Geometry: see drawing. Coordinates: mm, zero at the bounding-box minimum. Give positions to 0.01 mm unless a question says otherwise; leave off trailing zeros. Write each loop counter-clockwise with the first axis right and the second up, starting at its lowest first coordinate (ties: lowest second). Pieces come first, ordered by that corner, then holes. Notation, with made-up numbers: (-36, 10) - (-26, 10) arc R21 ccw to (-26, 43) - close; hole circle Ø1 at (7, -5). An arc over 180 degrees is marked (long way). Use a Markdown table: item, result. Add a question column.
1. Pin query (flat end, axial travel): pin 1 (3 mm diameter, centred on y = 86, z = 2, fed in from -X). Return the tip coordinate at first contact, or that it passes through.
2. Material intervals for probe 1 along X at (y, z) = (81.5, 5.5); probe 2 along Y at (x, z) = (42, 3.5) (1 decimal); probe 3 along X at (y, z) = (75, 6.25) (1 decimal), sorted ascending.
3. Section query A-A, the plane y = 79.5. Return loops of the section in (x, z).
4. Section query C-C, the plane z = 4.5. Return loops of the section in (x, y).
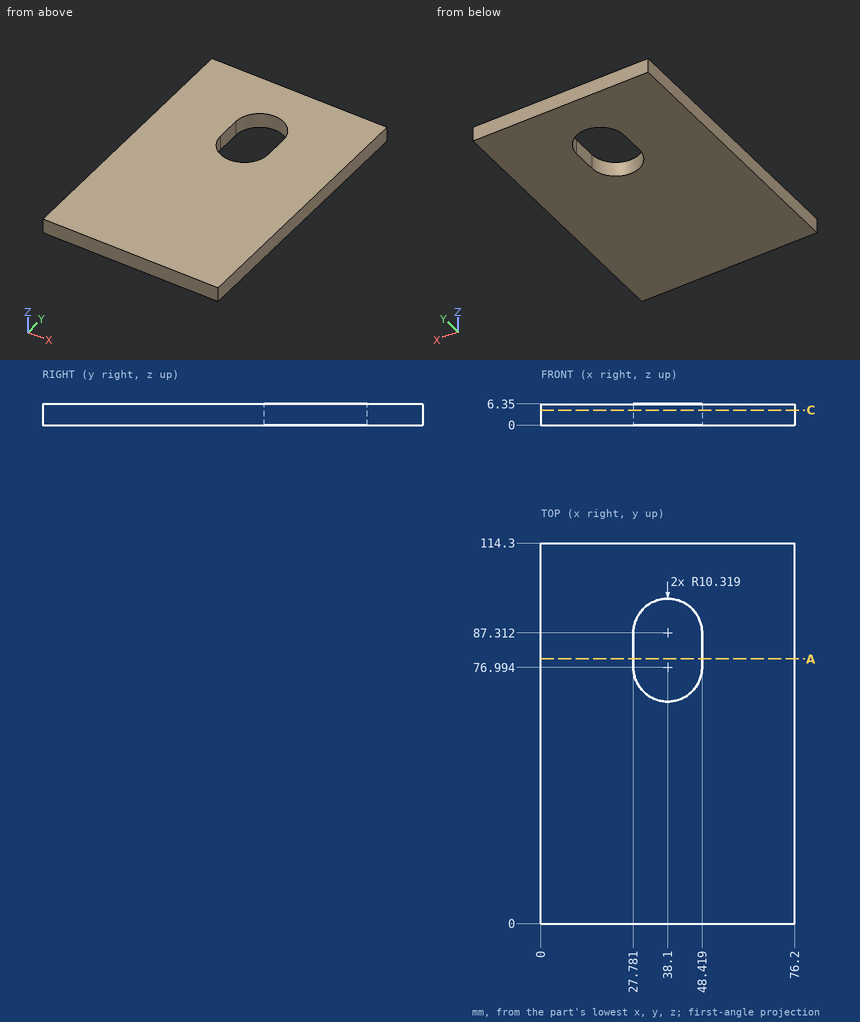
Result sheet:
| question | item | result |
|---|---|---|
| 1 | pin 1 | stops at x = 0 |
| 2 | probe 1 | x = 0 to 27.78, 48.42 to 76.2 |
| 2 | probe 2 | y = 0 to 67.4, 96.9 to 114.3 |
| 2 | probe 3 | x = 0 to 28, 48.2 to 76.2 |
| 3 | outline | (0, 0) - (27.78, 0) - (27.78, 6.35) - (0, 6.35) - close; (48.42, 0) - (76.2, 0) - (76.2, 6.35) - (48.42, 6.35) - close |
| 4 | outline | (0, 0) - (76.2, 0) - (76.2, 114.3) - (0, 114.3) - close; hole (27.78, 76.99) arc R10.32 ccw to (48.42, 76.99) - (48.42, 87.31) arc R10.32 ccw to (27.78, 87.31) - close |
